from build123d import *

# Parameters (mm, degrees)
F0_W          = 25.4
F0_H          = 25.4
F1_DEPTH      = 3.175
F1_TAPER      = -3
F3_W          = 2.9493607581
F3_H          = 9.1879377142
F6_DEPTH      = 4.5939688571
F6_DEPTH_BACK = 4.5939688571
F7_R          = 5.08


with BuildPart() as f1:
    # F0 (on Top) → F1 (new body)
    with BuildSketch(Plane.XY):
        Rectangle(F0_W, F0_H)
    extrude(amount=F1_DEPTH, taper=F1_TAPER)

    # F4: sweep along a path in F2
    with BuildLine(Plane.XZ) as f4_path:
        ThreePointArc((-10.16, 0), (0, -23.5582897328), (10.16, 0))
    # F3 (on face) → F4 (sweep)
    with BuildSketch(Plane.XY):
        with Locations((10.1631330326, 0)):
            Rectangle(F3_W, F3_H)
    sweep(path=f4_path.line)

    # F5 (on Front) → F6 (join, two sides)
    with BuildSketch(Plane.XZ) as f6_sk:
        with BuildLine():
            Line((-10.16, 0), (-10.0748691618, -1.4690828204))
            ThreePointArc((-10.0748691618, -1.4690828204), (-9.4103726, -0.7074453448), (-8.6884526536, 0))
            Line((-8.6884526536, 0), (-10.16, 0))
        make_face()
    extrude(amount=F6_DEPTH)
    extrude(f6_sk.sketch, amount=-F6_DEPTH_BACK)

    # F7
    f7_edges = [f1.edges().sort_by_distance(p)[0] for p in [
        (-12.783197, 12.783197, 1.5875),
        (-12.783197, -12.783197, 1.5875),
        (12.783197, -12.783197, 1.5875),
        (12.783197, 12.783197, 1.5875),
    ]]
    fillet(f7_edges, radius=F7_R)


solid = f1.part
Can you work these out from the model? Positions are in its coordinate system, mm. A direction names the side the tool comes from. Give positions to 0.01 mm unless a question says otherwise; leave off trailing zeros. Order: outer loops, then holes, each group sorted by start corner. A loop starts at its lowest first (then second) coordinate and runs counter-clockwise, first axis right, second up. Notation, with made-up numbers: (79.5, 58.25) - (97.5, 58.25) arc R26 ccw to (97.5, 95.25) - close; hole circle Ø1 at (75.25, 10.5). An arc over 180 degrees is marked (long way). Write each question's results on one line, items separated by ' | '.
1) Suppose I cut it at A-A, the plane z = -3. Write out the boundary of the cut face in (x, y), then the cut area to 3 significant figures.
Final values:
outline: (-13.56, -4.59) - (-11.14, -4.59) - (-11.14, 4.59) - (-13.56, 4.59) - close; (11.14, -4.59) - (13.56, -4.59) - (13.56, 4.59) - (11.14, 4.59) - close | area: 44.6 mm^2
2) Please list where these lines run through material, in increasing order: line 1 along Z through (x, y) = (0, -1.5) (3 decimals); line 2 along X through (y, z) = (2.5, -9.75); line 3 along Y through (x, z) = (12.5, -4.5). Write a range as [from, to].
Final values:
line 1: z = [-24.667, -22.528], [0, 3.175] | line 2: x = [-15.08, -12.94], [12.94, 15.08] | line 3: y = [-4.59, 4.59]
3) If we mould it in two halves opening along X, with no side actions, what happens to faces 4 (the face through (0, 0, 3.175)), 5 (the face through (0, 0, 0))? For each: pulls with the +X half, pulls with the -X half, needs draft (parallel to the pull), parting line crosses it, or undercut.
Final values:
face 4: needs draft | face 5: undercut
4) I'm going to push flat-ended pins straight in: pin 1 Ø6 at (x, y) = (-8.5, -10) entering from -Z; pin 2 Ø6 at (x, z) = (-1, -17.5) entering from +Y; pin 3 Ø6 at (y, z) = (3.5, -3.5) entering from -X; pin 4 Ø2 at (y, z) = (-3.5, -2) entering from -X. Where does each tip first touch, or does it pass through?
Final values:
pin 1: stops at z = 0 | pin 2: passes through | pin 3: stops at x = -14.76 | pin 4: stops at x = -13.56
5) Suppose I cut it at B-B, the plane z = -20. Write out the boundary of the cut face in (x, y).
Final values:
outline: (-10.91, -4.59) - (-7.68, -4.59) - (-7.68, 4.59) - (-10.91, 4.59) - close; (7.68, -4.59) - (10.91, -4.59) - (10.91, 4.59) - (7.68, 4.59) - close
6) On a 3-axis mill with a long thin cutter (end or side, diameter ignored), from which of +Z, -Z, +X, -X, +Y, -Y can I reach the whole of each face in a straight line? I mean faces 1 (the face through (3.3, -4.594, -22.3)), 2 (the face through (0.44, -0.06, -22.52)), 3 (the face through (3.3, 4.594, -22.3)). Say none if no direction works.
Final values:
face 1: -Z, +X, -X, -Y | face 2: +Y, -Y | face 3: -Z, +X, -X, +Y
